```python
from build123d import *

# Parameters (mm, degrees)
SKETCH1_R           = 1.5
SKETCH1_R_2         = 11
SKETCH1_R_3         = 2
BOSS_EXTRUDE1_DEPTH = 7
CUT_EXTRUDE1_DEPTH  = 4.5
SKETCH3_W           = 33.429321272
SKETCH3_H           = 5.85707368
CUT_EXTRUDE2_DEPTH  = 4.5
CHAMFER1_SIZE       = 3


with BuildPart() as part:
    # Sketch1 → Boss-Extrude1 (new body)
    with BuildSketch(Plane(origin=(0, 0, 0), x_dir=(0, 0, -1), z_dir=(1, 0, 0))):
        with BuildLine():
            Line((10.478493311, 20.815789474), (19, 20.815789474))
            Line((19, 20.815789474), (19, -19.184210526))
            Line((19, -19.184210526), (-19, -19.184210526))
            Line((-19, -19.184210526), (-19, 20.815789474))
            Line((-19, 20.815789474), (-1.478493311, 20.815789474))
            ThreePointArc((-1.478493311, 20.815789474), (4.5, 23.5), (10.478493311, 20.815789474))
        make_face()
        with Locations((15.5, -15.5)):
            Circle(SKETCH1_R, mode=Mode.SUBTRACT)
        with Locations((-15.5, 15.5)):
            Circle(SKETCH1_R, mode=Mode.SUBTRACT)
        with Locations((-15.5, -15.5)):
            Circle(SKETCH1_R, mode=Mode.SUBTRACT)
        Circle(SKETCH1_R_2, mode=Mode.SUBTRACT)
        with Locations((4.5, 15.5)):
            Circle(SKETCH1_R_3, mode=Mode.SUBTRACT)
    extrude(amount=BOSS_EXTRUDE1_DEPTH)

    # Sketch2 → Cut-Extrude1 (cut)
    with BuildSketch(Plane.ZY):
        with BuildLine():
            Line((-17.5, -13), (-17.5, 18.815789474))
            Line((-17.5, 18.815789474), (13, 18.815789474))
            Line((13, 18.815789474), (13, 15.5))
            ThreePointArc((13, 15.5), (13.732233047, 13.732233047), (15.5, 13))
            Line((15.5, 13), (17.5, 13))
            Line((17.5, 13), (17.5, -13))
            Line((17.5, -13), (15.5, -13))
            ThreePointArc((15.5, -13), (13.732233047, -13.732233047), (13, -15.5))
            Line((13, -15.5), (13, -17.684210526))
            Line((13, -17.684210526), (-13, -17.684210526))
            Line((-13, -17.684210526), (-13, -15.5))
            ThreePointArc((-13, -15.5), (-13.732233047, -13.732233047), (-15.5, -13))
            Line((-15.5, -13), (-17.5, -13))
        make_face()
    extrude(amount=-CUT_EXTRUDE1_DEPTH, mode=Mode.SUBTRACT)

    # Sketch3 → Cut-Extrude2 (cut)
    with BuildSketch(Plane.ZY):
        with Locations((-7.214660636, 21.744326314)):
            Rectangle(SKETCH3_W, SKETCH3_H)
    extrude(amount=-CUT_EXTRUDE2_DEPTH, mode=Mode.SUBTRACT)

    # Chamfer1
    chamfer1_edges = [part.edges().sort_by_distance(p)[0] for p in [
        (3.5, -19.184210526, -19),
        (3.5, -19.184210526, 19),
        (3.5, 20.815789474, 19),
        (5.75, 20.815789474, -19),
    ]]
    chamfer(chamfer1_edges, length=CHAMFER1_SIZE)


solid = part.part
```
Geometry: final body of the model. Coordinates: model frame, mm. A direction names the side the tool comes from. Round coordinates to 2 decimals unless told otherwise and drop trailing zeros. Order: outer loops, then holes, each group sorted by start corner. A loop starts at its lowest first (then second) coordinate and runs counter-clockwise, first axis right, second up. Notation, with made-up numbers: (66, 18.25) - (96, 18.25) arc R5 ccw to (96, 24.25) - close; hole circle Ø4 at (87.5, 35). An arc over 180 degrees is marked (long way). Write item = value, one per line. Start each with the question number.
Q1. Cut plane D-D on x = 5.5. Return the cut outline in (y, z).
Q2. Access query for faces 1 (the flat face through (2, 18.816, 11)), 2 (the flat face through (4, 20.816, 10)), 3 (the flat face through (7, 7, -9)), 4 (the flat face through (3, 1, 19)), 5 (the flat face through (2, -17, -13)). Directions: +Z, -Z, +X, -X, +Y, -Y. A direction counts if a zero-diameter tool reaches every point of the face in a straight line with its end or side. Return the directions, or none.
Q3. Cut plane C-C on z = 2. Return the cut outline in (x, y).
Q4. Ray query, line 1 (Y direction, x = 4.75, z = 15.5); line 2 (Z direction, x = 6.2, y = 0); line 3 (Z direction, x = 4.25, y = -5). Return the intervals inside material, ascending. Write a range as from..to.
Q5. Pin query (flat end, axial travel): pin 1 (3.5 mm diameter, centred on x = 1.5, z = 3, fed in from +Y); pin 2 (2 mm diameter, centred on x = 5, z = 8.5, fed in from +Y); pin 3 (1.6 mm diameter, centred on x = 3, y = 20, fed in from -Z). Return the tip coordinate at first contact, or that it passes through.
Q6. Pull-direction query (Y, two-part tool) for faces 6 (the flat face through (2, -13, 17)), 7 (the flat face through (2, 20, 9.5)), 8 (the flat face through (2, -13, -16)); classes: +Y half, -Y half, draft (parallel to the pull), parting line (faces both ways), or undercut.
Q7. Cut plane A-A on y = 0. Return the cut outline in (x, z), and give its area (3 significant figures).
Q8. Cut plane B-B on x = 1. Return the cut outline in (y, z), and give its area (3 significant figures).
Outcome:
q1.outline = (-19.18, -16) - (-16.18, -19) - (17.82, -19) - (20.82, -16) - (20.82, -10.48) arc R8 ccw to (20.82, 1.48) - (20.82, 16) - (17.82, 19) - (-16.18, 19) - (-19.18, 16) - close; hole circle Ø3 at (-15.5, -15.5); hole circle Ø3 at (-15.5, 15.5); hole circle Ø22 at (0, 0); hole circle Ø4 at (15.5, -4.5); hole circle Ø3 at (15.5, 15.5)
q2.face_1 = -X
q2.face_2 = +Z, +X, -X, +Y
q2.face_3 = +Z, -Z, +X, +Y, -Y
q2.face_4 = +Z, +X, -X, +Y, -Y
q2.face_5 = -X, +Y
q3.outline = (0, -19.18) - (7, -19.18) - (7, -10.82) - (4.5, -10.82) - (4.5, -17.68) - (0, -17.68) - close; (4.5, 10.82) - (7, 10.82) - (7, 20.82) - (4.5, 20.82) - close
q4.line_1 = -19.18..-17, -14..14, 17..20.82
q4.line_2 = -19..-11, 11..19
q4.line_3 = -19..-17.5, 17.5..19
q5.pin_1 = -17.68
q5.pin_2 = 20.82
q5.pin_3 = 9.5
q6.face_6 = undercut
q6.face_7 = draft
q6.face_8 = +Y half
q7.outline = (0, -19) - (7, -19) - (7, -11) - (4.5, -11) - (4.5, -17.5) - (0, -17.5) - close; (0, 17.5) - (4.5, 17.5) - (4.5, 11) - (7, 11) - (7, 19) - (0, 19) - close
q7.area = 53.5 mm^2
q8.outline = (-19.18, -16) - (-16.18, -19) - (17.82, -19) - (18.82, -18) - (18.82, -17.5) - (-13, -17.5) - (-13, -15.5) arc R2.5 ccw to (-15.5, -13) - (-17.68, -13) - (-17.68, 13) - (-15.5, 13) arc R2.5 ccw to (-13, 15.5) - (-13, 17.5) - (13, 17.5) - (13, 15.5) arc R2.5 ccw to (15.5, 13) - (18.82, 13) - (18.82, 9.5) - (20.82, 9.5) - (20.82, 16) - (17.82, 19) - (-16.18, 19) - (-19.18, 16) - close; hole circle Ø3 at (-15.5, -15.5); hole circle Ø3 at (-15.5, 15.5); hole circle Ø3 at (15.5, 15.5)
q8.area = 215 mm^2
